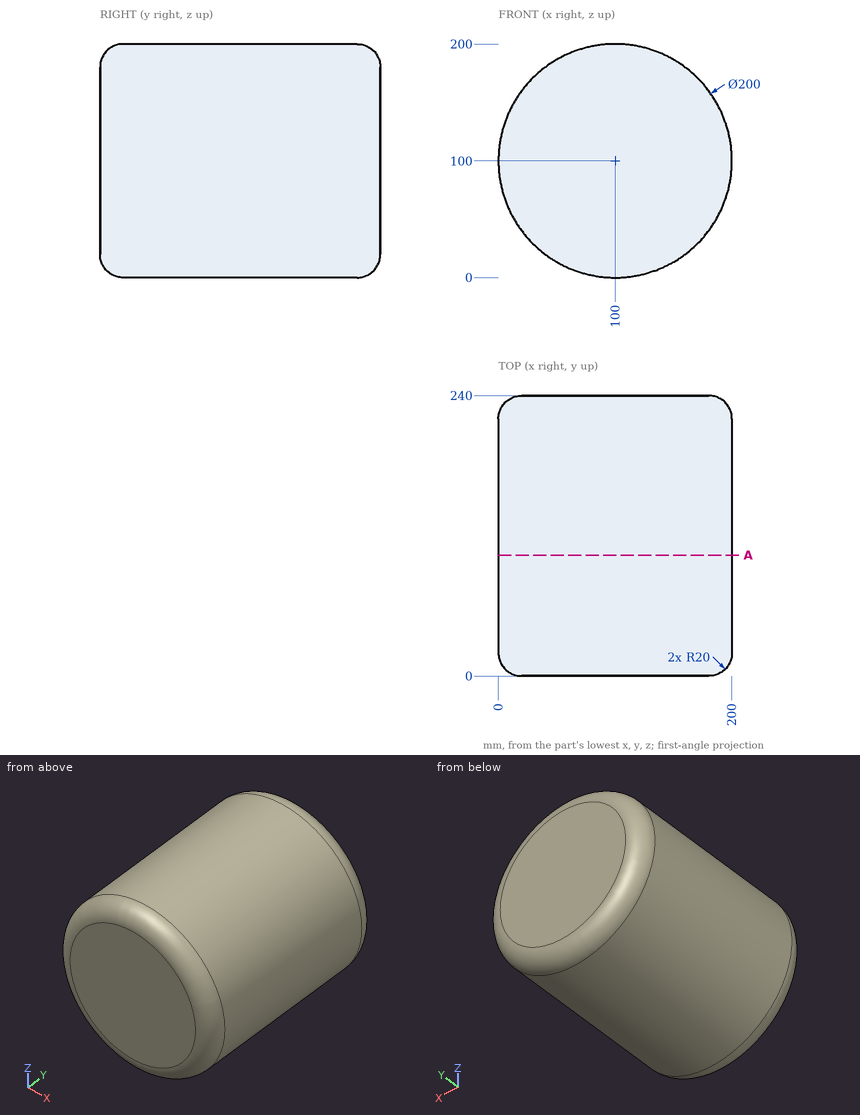
Here's the drawing with two shaded views (mm, measured from the low corner). I have some questions. Round coordinates to 2 decimals unless told otherwise and drop trailing zeros. Loops run counter-clockwise (first coordinate to the right, second up) from the corner with the lowest first, then second, coordinate; pieces in that order, holes last. Notation, with made-up numbers: M 25.5,89.5 L 51.5,89.5 A18 ccw 51.5,94.5 Z; hole C 83.25,88 d6. An arc over 180 degrees is marked long. Put each result on its own line as item: value.
Q1. For pin 1 (5 mm diameter, centred on y = 37, z = 93, fed in from -X); pin 2 (5 mm diameter, centred on x = 139.5, y = 52.5, fed in from -Z); pin 3 (3 mm diameter, centred on x = 75.5, y = 77.5, fed in from -Z), each with a flat end and sliding along its axis, tell me the tip position at first contact or that it passes through.
Check result:
pin 1: x = 0.1
pin 2: z = 7.1
pin 3: z = 2.68
Q2. Imagine slicing it at A-A (y = 103.5). Write out the boundary of the cut face in (x, z), then the cut area to 3 significant figures.
Check result:
outline: C 100,100 d200
area: 31,400 mm2
Q3. I need wall thicknesses on probe 1 along X at (y, z) = (60.5, 139); probe 2 along X at (y, z) = (117, 9.5); probe 3 along Z at (x, y) = (104.5, 120.5). Which ranges of each line are inside material? Lowest first, please.
Check result:
probe 1: 7.92 to 192.08
probe 2: 57.46 to 142.54
probe 3: 0.1 to 199.9
